Read the model definition and answer for the solid it produces. Units are mm, in the model's axes. Coordinates: 2 decimals unless noted, no trailing zeros. Loops run counter-clockwise (first coordinate to the right, second up) from the corner with the lowest first, then second, coordinate; pieces in that order, holes last. Notation, with made-up numbers: (-11.5, 65.25) -> (19.5, 65.25) arc R9 ccw to (19.5, 73.25) -> close; hole circle Ø5 at (81.25, 88.25). An arc over 180 degrees is marked (long way). Answer as CSV lines item,"result".
Autodesk Inventor part; units mm, degrees
ref_plane "YZ Plane" through (0, 0, 0) normal (1, 0, 0) x (0, 1, 0)
ref_plane "XZ Plane" through (0, 0, 0) normal (0, 1, 0) x (-1, 0, 0)
ref_plane "XY Plane" through (0, 0, 0) normal (0, 0, 1) x (1, 0, 0)
sketch "Sketch5" plane through (0, 0, 0) normal (0, 0, 1) x (1, 0, 0)
  line L0 (750, 1000) -> (-750, 1000)
  line L1 (-750, 1000) -> (-750, -1000)
  line L2 (-750, -1000) -> (750, -1000)
  line L3 (750, -1000) -> (750, 1000)
  line L4 (750, 1000) -> (-750, -1000) construction
  line L5 (-750, 1000) -> (750, -1000) construction
  line L6 (726, 976) -> (-726, 976)
  line L7 (-726, 976) -> (-726, -976)
  line L8 (-726, -976) -> (726, -976)
  line L9 (726, -976) -> (726, 976)
  line L10 (726, 976) -> (-726, -976) construction
  line L11 (-726, 976) -> (726, -976) construction
  point P0 (0, 0)
  dimension "d14" = 2000
  dimension "d15" = 1500
  dimension "d16" = 24
  dimension "d17" = 24
extrude "Extrusion4" add sketch "Sketch5" along normal blind 48
sketch "Sketch6" plane through (0, 0, 48) normal (0, 0, 1) x (1, 0, 0)
  line L0 (-750, 1000) -> (-750, -1000) construction
  line L1 (-750, -1000) -> (750, -1000) construction
  line L2 (750, -1000) -> (750, 1000) construction
  line L3 (750, 1000) -> (-750, 1000) construction
  line L4 (726, 976) -> (726, -976) construction
  line L5 (726, -976) -> (-726, -976) construction
  line L6 (-726, -976) -> (-726, 976) construction
  line L7 (-726, 976) -> (726, 976) construction
  line L8 (750, -1000) -> (702, -1000)
  line L9 (702, -1000) -> (702, -976)
  line L10 (702, -976) -> (750, -976)
  line L11 (750, -976) -> (750, -1000)
  line L12 (-750, -1000) -> (-702, -1000)
  line L13 (-702, -1000) -> (-702, -976)
  line L14 (-702, -976) -> (-750, -976)
  line L15 (-750, -976) -> (-750, -1000)
  line L16 (-750, 1000) -> (-702, 1000)
  line L17 (-702, 1000) -> (-702, 976)
  line L18 (-702, 976) -> (-750, 976)
  line L19 (-750, 976) -> (-750, 1000)
  line L20 (750, 1000) -> (702, 1000)
  line L21 (702, 1000) -> (702, 976)
  line L22 (702, 976) -> (750, 976)
  line L23 (750, 976) -> (750, 1000)
  point P0 (0, 0)
  dimension "d20" = 48
  dimension "d21" = 48
extrude "Extrusion5" add sketch "Sketch6" along normal blind 1500
sketch "Sketch7" plane through (0, 0, 1548) normal (0, 0, 1) x (1, 0, 0)
  line L0 (-702, -976) -> (-702, -1000) construction
  line L1 (-702, -1000) -> (702, -1000) construction
  line L2 (702, -1000) -> (702, -976) construction
  line L3 (702, -976) -> (-702, -976) construction
  line L4 (-726, 976) -> (-750, 976) construction
  line L5 (-750, 976) -> (-750, -976) construction
  line L6 (-750, -976) -> (-726, -976) construction
  line L7 (-726, -976) -> (-726, 976) construction
  line L8 (702, 1000) -> (702, 976) construction
  line L9 (702, 976) -> (750, 976) construction
  line L10 (750, 976) -> (750, 1000) construction
  line L11 (750, 1000) -> (702, 1000) construction
  line L12 (750, 1000) -> (-750, 1000)
  line L13 (-750, 1000) -> (-750, -1000)
  line L14 (-750, -1000) -> (750, -1000)
  line L15 (750, -1000) -> (750, 1000)
  line L16 (-726, -976) -> (726, -976)
  line L17 (726, -976) -> (726, 976)
  line L18 (726, 976) -> (-726, 976)
  line L19 (-726, 976) -> (-726, -976)
  point P0 (0, 0)
  dimension "d24" = 24
extrude "Extrusion6" add sketch "Sketch7" along normal blind 48
sketch "Sketch8" plane through (750, -1000, 0) normal (1, 0, 0) x (0, 0, -1)
  line L0 (-48, 1976) -> (-1548, 1976) construction
  line L1 (-48, 24) -> (-48, 1976) construction
  line L2 (-48, 24) -> (-1548, 24) construction
  line L3 (-1548, 24) -> (-1548, 1976) construction
  line L4 (0, 2000) -> (-1596, 2000) construction
  line L5 (-1596, 0) -> (-1596, 2000) construction
  line L6 (0, 0) -> (-1596, 0) construction
  line L7 (0, 0) -> (0, 2000) construction
  line L8 (-1596, 0) -> (0, 0)
  line L9 (0, 0) -> (0, 2000)
  line L10 (0, 2000) -> (-1596, 2000)
  line L11 (-1596, 2000) -> (-1596, 0)
  point P0 (0, 1000)
extrude "Extrusion7" add sketch "Sketch8" along normal blind 0.1
sketch "Sketch9" plane through (-750, -1000, 0) normal (0, -1, 0) x (1, 0, 0)
  line L0 (1452, 48) -> (1452, 1548) construction
  line L1 (48, 48) -> (1452, 48) construction
  line L2 (48, 48) -> (48, 1548) construction
  line L3 (48, 1548) -> (1452, 1548) construction
  line L4 (0, 1596) -> (1500.1, 1596) construction
  line L5 (0, 0) -> (0, 1596) construction
  line L6 (0, 0) -> (1500.1, 0) construction
  line L7 (1500.1, 1596) -> (1500.1, 0) construction
  line L8 (0, 1596) -> (1500.1, 1596)
  line L9 (1500.1, 1596) -> (1500.1, 0)
  line L10 (1500.1, 0) -> (0, 0)
  line L11 (0, 0) -> (0, 1596)
  point P0 (750, 0)
extrude "Extrusion8" add sketch "Sketch9" along normal blind 0.1
sketch "Sketch10" plane through (-750, 1000, 0) normal (-1, 0, 0) x (0, 0, 1)
  line L0 (0, 0) -> (1596, 0) construction
  line L1 (0, 0) -> (0, -2000.1) construction
  line L2 (1596, -2000.1) -> (0, -2000.1) construction
  line L3 (1596, 0) -> (1596, -2000.1) construction
  line L4 (1548, -24) -> (1548, -1976) construction
  line L5 (48, -1976) -> (1548, -1976) construction
  line L6 (48, -24) -> (48, -1976) construction
  line L7 (48, -24) -> (1548, -24) construction
  line L8 (1596, 0) -> (0, 0)
  line L9 (0, 0) -> (0, -2000.1)
  line L10 (0, -2000.1) -> (1596, -2000.1)
  line L11 (1596, -2000.1) -> (1596, 0)
  line L12 (1348, -700) -> (1048, -700)
  line L13 (1048, -700) -> (1048, -1300)
  line L14 (1048, -1300) -> (1348, -1300)
  line L15 (1348, -1300) -> (1348, -700)
  line L16 (-319.34, -1000) -> (1915.34, -1000) construction
  point P0 (0, -1000)
  dimension "d37" = 600
  dimension "d38" = 300
  dimension "d39" = 300
  dimension "d40" = 1000
extrude "Extrusion9" add sketch "Sketch10" along normal blind 0.1
sketch "Sketch11" plane through (0, 0, 1596) normal (0, 0, 1) x (1, 0, 0)
  line L0 (750.1, -1000.1) -> (-750.1, -1000.1) construction
  line L1 (750.1, 1000) -> (750.1, -1000.1) construction
  line L2 (-750.1, 1000) -> (750.1, 1000) construction
  line L3 (-750.1, -1000.1) -> (-750.1, 1000) construction
  line L4 (-726, -976) -> (-726, 976) construction
  line L5 (-726, 976) -> (726, 976) construction
  line L6 (726, 976) -> (726, -976) construction
  line L7 (726, -976) -> (-726, -976) construction
  line L8 (750.1, 1000) -> (-750.1, 1000)
  line L9 (-750.1, 1000) -> (-750.1, -1000.1)
  line L10 (-750.1, -1000.1) -> (750.1, -1000.1)
  line L11 (750.1, -1000.1) -> (750.1, 1000)
  point P0 (0, 0)
extrude "Extrusion10" add sketch "Sketch11" along normal blind 0.1
sketch "Sketch12" plane through (0, 0, 0) normal (0, 0, -1) x (-1, 0, 0)
  line L0 (750.1, 1000) -> (-750.1, 1000) construction
  line L1 (-750.1, 1000) -> (-750.1, -1000.1) construction
  line L2 (-750.1, -1000.1) -> (750.1, -1000.1) construction
  line L3 (750.1, 1000) -> (750.1, -1000.1) construction
  line L4 (-726, 976) -> (-726, -976) construction
  line L5 (726, 976) -> (-726, 976) construction
  line L6 (726, -976) -> (726, 976) construction
  line L7 (-726, -976) -> (726, -976) construction
  line L8 (750.1, 1000) -> (-750.1, 1000)
  line L9 (-750.1, 1000) -> (-750.1, -1000.1)
  line L10 (-750.1, -1000.1) -> (750.1, -1000.1)
  line L11 (750.1, -1000.1) -> (750.1, 1000)
  point P0 (0, 0)
extrude "Extrusion11" add sketch "Sketch12" along normal blind 0.1
sketch "Sketch13" plane through (-750.1, 1000, 1596.1) normal (0, 1, 0) x (1, 0, 0)
  line L0 (48.1, 1548.1) -> (48.1, 48.1) construction
  line L1 (1452.1, 1548.1) -> (48.1, 1548.1) construction
  line L2 (1452.1, 1548.1) -> (1452.1, 48.1) construction
  line L3 (1452.1, 48.1) -> (48.1, 48.1) construction
  line L4 (1500.2, 0) -> (1500.2, 1596.2) construction
  line L5 (0, 1596.2) -> (1500.2, 1596.2) construction
  line L6 (0, 1596.2) -> (0, 0) construction
  line L7 (1500.2, 0) -> (0, 0) construction
  line L8 (0, 0) -> (1500.2, 1596.2)
  line L9 (1500.2, 0) -> (1500.2, 1596.2)
  line L10 (1500.2, 0) -> (0, 0)
  point P0 (750.1, 1596.1)
extrude "Extrusion12" add sketch "Sketch13" along normal blind 0.1
properties part number "P004_CageDeTest2"
Q1. A cutting plane is placed at D-D, the plane x = 485. Write down the section's boundary in (y, z), and give its area (3 significant figures).
Results:
outline,"(-1000.1, -0.1) -> (1000, -0.1) -> (1000, 48) -> (976, 48) -> (976, 0) -> (-976, 0) -> (-976, 48) -> (-1000, 48) -> (-1000, 1548) -> (-976, 1548) -> (-976, 1596) -> (976, 1596) -> (976, 1548) -> (1000, 1548) -> (1000, 281.96) -> (1000.1, 281.96) -> (1000.1, 1596.1) -> (-1000.1, 1596.1) -> close"
area,"5,300 mm²"
Q2. A cutting plane is placed at A-A, the plane y = 427.5. Write down the section's boundary in (x, z).
Results:
outline,"(-750.1, -0.1) -> (750.1, -0.1) -> (750.1, 1596.1) -> (-750.1, 1596.1) -> close; hole (-750, 48) -> (-726, 48) -> (-726, 0) -> (726, 0) -> (726, 48) -> (750, 48) -> (750, 1548) -> (726, 1548) -> (726, 1596) -> (-726, 1596) -> (-726, 1548) -> (-750, 1548) -> close"
Q3. A cutting plane is placed at C-C, the plane z = 1140. Write down the section's boundary in (x, y).
Results:
outline,"(-750.1, -1000.1) -> (750.1, -1000.1) -> (750.1, 1000.1) -> (-321.43, 1000.1) -> (-321.43, 1000) -> (702, 1000) -> (702, 976) -> (750, 976) -> (750, -976) -> (702, -976) -> (702, -1000) -> (-702, -1000) -> (-702, -976) -> (-750, -976) -> (-750, -300) -> (-750.1, -300) -> close; (-750.1, 300) -> (-750, 300) -> (-750, 976) -> (-702, 976) -> (-702, 1000) -> (-750.1, 1000) -> close"
Q4. Given pin 1 Ø3 at (x, z) = (-272, 257.5) entering from +Y, flat-ended and moving along its own axis, determine where the tip first touches the part or whether it passes through.
Results:
pin 1,"stops at y = -1000"
Q5. A cutting plane is placed at B-B, the plane y = -138. Write down the section's boundary in (x, z), and give its area (3 significant figures).
Results:
outline,"(-750.1, -0.1) -> (750.1, -0.1) -> (750.1, 1596.1) -> (-750.1, 1596.1) -> (-750.1, 1348) -> (-750, 1348) -> (-750, 1548) -> (-726, 1548) -> (-726, 1596) -> (726, 1596) -> (726, 1548) -> (750, 1548) -> (750, 48) -> (726, 48) -> (726, 0) -> (-726, 0) -> (-726, 48) -> (-750, 48) -> (-750, 1048) -> (-750.1, 1048) -> close"
area,"5,200 mm²"
Q6. For a pull along Z with two mould halves and no side action, classify faces 1 (the face through (726, 976, 794)), 2 (the face through (-337, 1000, 33)), 3 (the face through (726, -14, 24)) as pulls with the +Z half, pulls with the -Z half, needs draft (parallel to the pull), parting line crosses it, or undercut.
Results:
face 1,"undercut"
face 2,"needs draft"
face 3,"undercut"
